```python
from build123d import *

# Parameters (mm, degrees)
CIRCLE002_R      = 3
EXTRUDE002_DEPTH = 1
CIRCLE_R         = 1
EXTRUDE_DEPTH    = 11
CIRCLE001_R      = 2
EXTRUDE001_DEPTH = 10


with BuildPart() as ext_foot:
    # Circle002 → Extrude002 (new body)
    with BuildSketch(Plane.XY):
        Circle(CIRCLE002_R)
    extrude(amount=EXTRUDE002_DEPTH)


with BuildPart() as ext_inner:
    # Circle → Extrude (new body)
    with BuildSketch(Plane.XY):
        Circle(CIRCLE_R)
    extrude(amount=EXTRUDE_DEPTH)


with BuildPart() as anti_flex:
    # Circle001 → Extrude001 (new body)
    with BuildSketch(Plane.XY):
        Circle(CIRCLE001_R)
    extrude(amount=EXTRUDE001_DEPTH)

    # Cut: cut ext_inner
    add(ext_inner.part, mode=Mode.SUBTRACT)

    # Fusion: union ext_foot
    add(ext_foot.part)


solid = anti_flex.part
```
Geometry check sheet. Reference: the model listing, model coordinates, mm. A direction names the side the tool comes from. Coordinates: 2 decimals unless noted, no trailing zeros. Loops run counter-clockwise (first coordinate to the right, second up) from the corner with the lowest first, then second, coordinate; pieces in that order, holes last. Notation, with made-up numbers: (-14.75, 18.5) -> (13.25, 18.5) arc R25 cw to (13.25, 51.5) -> close; hole circle Ø10 at (27.25, -5). An arc over 180 degrees is marked (long way). Put each result on its own line as item: value.
1) Cross-section at A-A on y = 0. Record the boundary of the cut face in (x, z), plus the area to 3 significant figures.
Result set:
outline: (-3, 0) -> (3, 0) -> (3, 1) -> (2, 1) -> (2, 10) -> (1, 10) -> (1, 1) -> (-1, 1) -> (-1, 10) -> (-2, 10) -> (-2, 1) -> (-3, 1) -> close
area: 24.0 mm^2
2) Cross-section at D-D on y = -1.15. Record the boundary of the cut face in (x, z).
Result set:
outline: (-2.77, 0) -> (2.77, 0) -> (2.77, 1) -> (1.64, 1) -> (1.64, 10) -> (-1.64, 10) -> (-1.64, 1) -> (-2.77, 1) -> close
3) Thickness scan on line 1 (Y direction, x = 0, z = 6.5); line 2 (Z direction, x = -0.2, y = 0.45). Record the ranges inside material, lowest first.
Result set:
line 1: y = -2 to -1, 1 to 2
line 2: z = 0 to 1
4) Cross-section at C-C on z = 8. Record the boundary of the cut face in (x, y), plus the area to 3 significant figures.
Result set:
outline: circle Ø4 at (0, 0); hole circle Ø2 at (0, 0)
area: 9.42 mm^2
5) Release check for a two-part mould opening along Y. For faces 3 (the flat face through (0, 0, 1)), 4 (the cylindrical face through (0, -1, 5)), 5 (the cylindrical face through (-3, 0.1, 0.5)), 6 (the flat face through (1, -1, 10)) record: released by +Y, released by -Y, zero draft, split by the parting line, or undercut.
Result set:
face 3: undercut
face 4: undercut
face 5: split by the parting line
face 6: zero draft
6) Tool access check on faces 1 (the flat face through (0, 0, 0)), 2 (the flat face through (1, -2, 1)). Record the directions out of +Z, -Z, +X, -X, +Y, -Y that give a thin tool (end or side, any length) a straight path to the whole face; none if there is none.
Result set:
face 1: -Z, +X, -X, +Y, -Y
face 2: +Z
7) Gauge pin test, flat end, axial feed: pin 1 Ø3 at (x, y) = (0, 0) entering from -Z. Record the tip position at first contact, or that the pin passes through.
Result set:
pin 1: stops at z = 0
